Check sheet for the modelled part. Datum: model origin and axes. Units: mm. A direction names the side the tool comes from. Round coordinates to 2 decimals unless told otherwise and drop trailing zeros. Loops run counter-clockwise (first coordinate to the right, second up) from the corner with the lowest first, then second, coordinate; pieces in that order, holes last. Notation, with made-up numbers: (76, 1.25) - (109, 1.25) arc R22 cw to (109, 37.25) - close; hole circle Ø10 at (-34, 57). An arc over 180 degrees is marked (long way). Put each result on its own line as item: value.
```python
from build123d import *

# Parameters (mm, degrees)
SKETCH1_R           = 3.5
SKETCH1_R_2         = 2
BOSS_EXTRUDE1_DEPTH = 9
SKETCH2_R           = 11.2
CUT_EXTRUDE1_DEPTH  = 7.3
CUT_EXTRUDE2_REACH  = 42.316
SKETCH3_R           = 6


with BuildPart() as part:
    # Sketch1 → Boss-Extrude1 (new body)
    with BuildSketch(Plane(origin=(0, 0, 0), x_dir=(1, 0, 0), z_dir=(0, 1, 0))):
        with BuildLine():
            Line((-6, 37), (6, 37))
            Line((6, 37), (6, 12.925265955))
            ThreePointArc((6, 12.925265955), (14.25, 0), (6, -12.925265955))
            Line((6, -12.925265955), (6, -37))
            Line((6, -37), (-6, -37))
            Line((-6, -37), (-6, -12.925265955))
            ThreePointArc((-6, -12.925265955), (-14.25, 0), (-6, 12.925265955))
            Line((-6, 12.925265955), (-6, 37))
        make_face()
        with Locations(Location((0, 22.5, 0), (0, 0, 270))):
            Circle(SKETCH1_R, mode=Mode.SUBTRACT)
        with Locations(Location((0, 32.5, 0), (0, 0, 270))):
            Circle(SKETCH1_R_2, mode=Mode.SUBTRACT)
        with Locations(Location((0, -22.5, 0), (0, 0, 90))):
            Circle(SKETCH1_R, mode=Mode.SUBTRACT)
        with Locations(Location((0, -32.5, 0), (0, 0, 90))):
            Circle(SKETCH1_R_2, mode=Mode.SUBTRACT)
    extrude(amount=BOSS_EXTRUDE1_DEPTH)

    # Sketch2 → Cut-Extrude1 (cut)
    with BuildSketch(Plane(origin=(0, 9, 0), x_dir=(1, 0, 0), z_dir=(0, 1, 0))):
        with Locations(Location((0, 0, 0), (0, 0, 270))):
            Circle(SKETCH2_R)
    extrude(amount=-CUT_EXTRUDE1_DEPTH, mode=Mode.SUBTRACT)

    # Sketch3 → Cut-Extrude2 (cut, up to next)
    with BuildSketch(Plane(origin=(0, 1.7, 0), x_dir=(1, 0, 0), z_dir=(0, 1, 0)), mode=Mode.PRIVATE) as cut_extrude2_sk1:
        with Locations(Location((0, 0, 0), (0, 0, 270))):
            Circle(SKETCH3_R)
    cut_extrude2_tool1 = extrude(cut_extrude2_sk1.sketch, amount=-CUT_EXTRUDE2_REACH, mode=Mode.PRIVATE) & part.part
    add(cut_extrude2_tool1.solids().sort_by_distance((0, 1.7, 0))[0], mode=Mode.SUBTRACT)


solid = part.part
```
Item 1: Go/stop test with flat-tipped pins: pin 1 (3 mm diameter, centred on y = 6, z = 29.5, fed in from -X); pin 2 (2 mm diameter, centred on x = -8.5, y = 7, fed in from -Z); pin 3 (4 mm diameter, centred on y = 6.5, z = -11.5, fed in from -X). Record where each tip stops, or that it passes through.
Filled sheet:
pin 1: x = -6
pin 2: z = -12.12
pin 3: x = -10.62
Item 2: Section check A-A on z = -32.5. Enter the section's corners in (x, y), then the cut area to 3 significant figures.
Filled sheet:
outline: (-6, 0) - (-2, 0) - (-2, 9) - (-6, 9) - close; (2, 0) - (6, 0) - (6, 9) - (2, 9) - close
area: 72.0 mm²
Item 3: Thickness scan on line 1 (X direction, y = 3, z = 22.5); line 2 (Z direction, x = 1.75, y = 1.5); line 3 (Z direction, x = 0.75, y = 6). Record the ranges inside material, lowest first. Write a range as from..to.
Filled sheet:
line 1: -6..-3.5, 3.5..6
line 2: -37..-33.47, -31.53..-25.53, -19.47..-5.74, 5.74..19.47, 25.53..31.53, 33.47..37
line 3: -37..-34.35, -30.65..-25.92, -19.08..-11.17, 11.17..19.08, 25.92..30.65, 34.35..37
Item 4: Section check D-D on z = 0. Enter the section's corners in (x, y).
Filled sheet:
outline: (-14.25, 0) - (-6, 0) - (-6, 1.7) - (-11.2, 1.7) - (-11.2, 9) - (-14.25, 9) - close; (6, 0) - (14.25, 0) - (14.25, 9) - (11.2, 9) - (11.2, 1.7) - (6, 1.7) - close
Item 5: Tool access check on faces 4 (the flat face through (-6, 4, 25)), 5 (the flat face through (-6, 4, -25)), 6 (the flat face through (6, 4, -25)). Record the directions out of +Z, -Z, +X, -X, +Y, -Y that give a thin tool (end or side, any length) a straight path to the whole face; none if there is none.
Filled sheet:
face 4: +Z, -X, +Y, -Y
face 5: -Z, -X, +Y, -Y
face 6: -Z, +X, +Y, -Y
Item 6: Section check B-B on y = 5.75. Enter the section's corners in (x, z), then the cut area to 3 significant figures.
Filled sheet:
outline: (-6, -37) - (6, -37) - (6, -12.93) arc R14.25 ccw to (6, 12.93) - (6, 37) - (-6, 37) - (-6, 12.93) arc R14.25 ccw to (-6, -12.93) - close; hole circle Ø22.4 at (0, 0); hole circle Ø7 at (0, -22.5); hole circle Ø7 at (0, 22.5); hole circle Ø4 at (0, -32.5); hole circle Ø4 at (0, 32.5)
area: 698 mm²
Item 7: Section check C-C on x = 8.25. Enter the section's corners in (y, z), then the cut area to 3 significant figures.
Filled sheet:
outline: (0, -11.62) - (9, -11.62) - (9, -7.57) - (1.7, -7.57) - (1.7, 7.57) - (9, 7.57) - (9, 11.62) - (0, 11.62) - close
area: 98.5 mm²
Item 8: Release check for a two-part mould opening along Z. For faces 1 (the cylindrical face through (0.766, 4.437, 30.653)), 2 (the flat face through (-3, 9, 11)), 3 (the cylindrical face through (-14.25, 4.44, 0.23)) record: +Z half, -Z half, draft (parallel to the pull), parting line (faces both ways), or undercut.
Filled sheet:
face 1: undercut
face 2: draft
face 3: parting line
